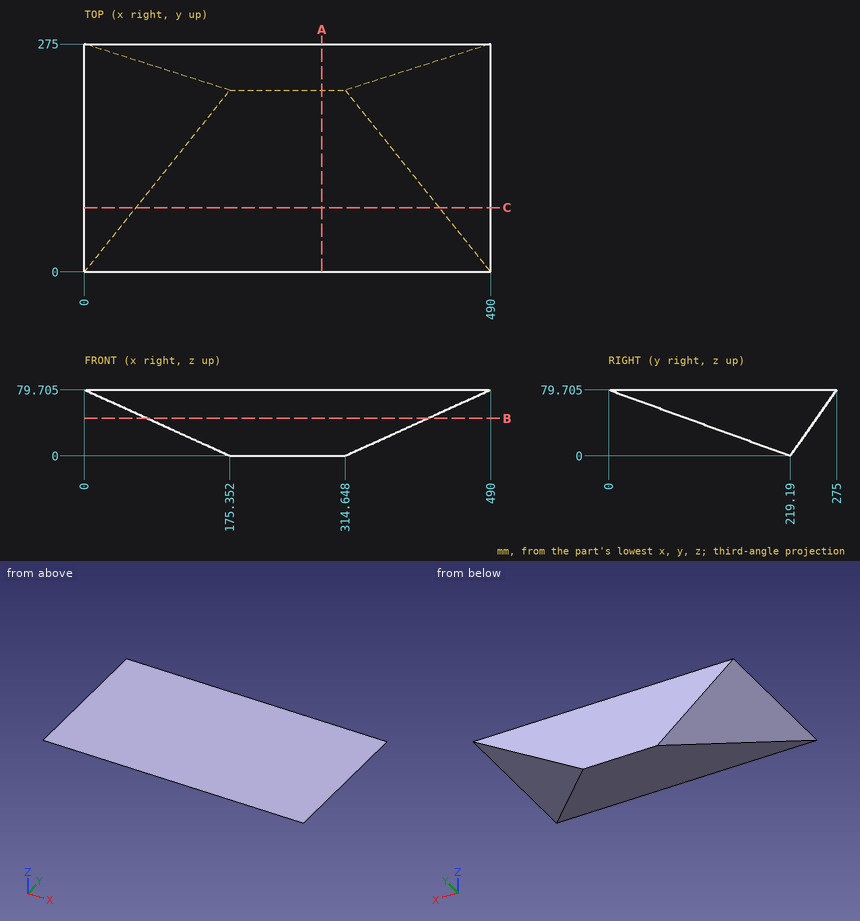
Design review of the part shown in the three views and the two pictorial views. Dimensions are in mm from the part's minimum x, y and z. Round coordinates to 2 decimals unless told otherwise and drop trailing zeros. Write each loop counter-clockwise with the first axis right and the second up, starting at its lowest first coordinate (ties: lowest second). Pieces come first, ordered by that corner, then holes. Notation, with made-up numbers: (-39, -27) - (-18, -27) arc R16 cw to (-18, -23) - close; hole circle Ø9 at (69.25, 58.5). An arc over 180 degrees is marked (long way). Return JSON: item names as keys, results as strings. Group by question number.
Item 1: Insertion check: P1, Ø3, axis at x = 359.5, z = 66, coming from the +Y side; P2, Ø2, axis at x = 331.5, z = 38.5, coming from the +Y side; P3, Ø3, axis at x = 205, z = 39.5, coming from the +Y side. Each pin has a flat end and moves straight along its axis. Give the tip position at first contact, or say it passes through.
Item 2: We need section C-C on y = 77.5. Write out the cut boundary in (x, z) (1 decimal).
Item 3: We need section A-A on x = 286.5. Write out the cut boundary in (y, z) (1 decimal), and give its area (3 significant figures).
Item 4: For probe 1 along Z at (x, y) = (52, 219) (1 decimal); probe 2 along Z at (x, y) = (90, 216) (1 decimal), list the stretches that pass through material, from the lowest coordinate up. Write a range as [from, to].
Item 5: We need section B-B on z = 45.5. Write out the cut boundary in (x, y) (1 decimal).
Model answer:
{
 "1": {"P1": "stops at y = 266.45", "P2": "stops at y = 246.85", "P3": "stops at y = 247.9"},
 "2": {"outline": "(0, 79.7) - (62, 51.5) - (428, 51.5) - (490, 79.7) - close"},
 "3": {"outline": "(0, 79.7) - (219.2, 0) - (275, 79.7) - close", "area": "11,000 mm²"},
 "4": {"probe 1": "z = [56.1, 79.7]", "probe 2": "z = [38.8, 79.7]"},
 "5": {"outline": "(75.3, 94.1) - (414.7, 94.1) - (414.7, 251) - (75.3, 251) - close"}
}
